Can you work these out from the model? Positions are in its coordinate system, mm. A direction names the side the tool comes from. Coordinates: 2 decimals unless noted, no trailing zeros. Order: outer loops, then holes, each group sorted by start corner. A loop starts at its lowest first (then second) coordinate and runs counter-clockwise, first axis right, second up. Notation, with made-up numbers: (85.25, 62.5) -> (122.25, 62.5) arc R30 cw to (122.25, 97.5) -> close; hole circle Ø6 at (9, 69). An arc over 180 degrees is marked (long way). Answer as a JSON object with one key per item and string values. Group by question number.
(1) I want a section at A-A, the plane x = -22. List the corners of the cut face in (y, z) for me.
(2) I need wall thicknesses on line 1 (X direction, y = 1, z = -5); line 2 (Y direction, x = -14, z = -10); line 3 (Z direction, x = 0, y = -1). Which ranges of each line are inside material? Lowest first, please.
(3) I want a section at D-D, the plane x = -47.5. List the corners of the cut face in (y, z) for me.
(4) Which directions (+Z, -Z, +X, -X, +Y, -Y) give clear straight access to the entire face, cutting with the end or side of a thin tool? Please do faces 5 (the flat face through (10.2, 1.844, 42.9)), 6 (the flat face through (7.5, 4.425, 44.7)), 7 (the flat face through (-37, -24.335, -13)), 8 (the flat face through (10.3, -4.425, 40.2)).
(5) For pin 1 (12 mm diameter, centred on x = -36, y = 27, fed in from +Z); pin 2 (3 mm diameter, centred on y = 27, z = -9, fed in from +X); pin 3 (2 mm diameter, centred on x = 11, z = 38, fed in from +Y); pin 4 (8 mm diameter, centred on y = -11, z = 5, fed in from +X), each with a flat end and sliding along its axis, tell me the tip position at first contact or that it passes through.
(6) I want a section at B-B, the plane y = -11. List the corners of the cut face in (x, z) for me.
(7) I want a section at C-C, the plane z = -18.5. List the corners of the cut face in (x, y) for me, plus the area to 3 significant figures.
(8) If we mould it in two halves opening along X, with no side actions, what happens to faces 1 (the flat face through (-29, 41.295, -13)), 2 (the cylindrical face through (11.815, -0.026, 46.62)), 3 (the flat face through (10.14, 0, -13)), 4 (the flat face through (-68.027, 0, -13))? For each: pulls with the +X half, pulls with the -X half, needs draft (parallel to the pull), parting line crosses it, or undercut.
from build123d import *

# Parameters (mm, degrees)
F0_W     = 14.748384
F0_H     = 8.849032
F0_W_2   = 7.005484
F0_H_2   = 3.687096
F3_W     = 78.166454
F3_H     = 82.406614
F3_W_2   = 44.982581
F3_H_2   = 48.669678
F4_DEPTH = 25.4
F5_DEPTH = 2.54


with BuildPart() as f2:
    # F2: sweep along a path in F1
    with BuildLine(Plane.XZ) as f2_path:
        ThreePointArc((0, 27.558451), (-16.169621, 43.728072), (-32.339242, 27.558451))
    # F0 (on Top) → F2 (sweep)
    with BuildSketch(Plane.XY):
        Rectangle(F0_W, F0_H)
        Rectangle(F0_W_2, F0_H_2, mode=Mode.SUBTRACT)
    sweep(path=f2_path.line)

    # F3 (on Top) → F4 (join)
    with BuildSketch(Plane.XY):
        with Locations((-28.943711, 0.092177)):
            Rectangle(F3_W, F3_H)
        with Locations((-36.317903, 0)):
            Rectangle(F3_W_2, F3_H_2, mode=Mode.SUBTRACT)
    extrude(amount=-F4_DEPTH)

    # F3 (on Top) → F5 (cut)
    with BuildSketch(Plane.XY):
        with Locations((-36.317903, 0)):
            Rectangle(F3_W_2, F3_H_2)
    extrude(amount=-F5_DEPTH, mode=Mode.SUBTRACT)


solid = f2.part
Computed values:
{
 "1": {"outline": "(-41.11, -25.4) -> (-24.33, -25.4) -> (-24.33, 0) -> (-41.11, 0) -> close; (-4.42, 55.89) -> (4.42, 55.89) -> (4.42, 63.33) -> (-4.42, 63.33) -> close; (24.33, -25.4) -> (41.3, -25.4) -> (41.3, 0) -> (24.33, 0) -> close; hole (-1.84, 57.32) -> (1.84, 57.32) -> (1.84, 60.91) -> (-1.84, 60.91) -> close"},
 "2": {"line 1": "x = -68.03 to -58.81, -13.83 to 10.14", "line 2": "y = -41.11 to -24.33, 24.33 to 41.3", "line 3": "z = -25.4 to 0, 1.9 to 3.57, 51.55 to 53.22, 57.31 to 60"},
 "3": {"outline": "(-41.11, -25.4) -> (-24.33, -25.4) -> (-24.33, 0) -> (-41.11, 0) -> close; (24.33, -25.4) -> (41.3, -25.4) -> (41.3, 0) -> (24.33, 0) -> close"},
 "4": {"face 5": "none", "face 6": "+Z, +X, -X, +Y", "face 7": "+Z, -Z", "face 8": "+Z, +X, -X, -Y"},
 "5": {"pin 1": "stops at z = 0", "pin 2": "stops at x = 10.14", "pin 3": "stops at y = 4.42", "pin 4": "passes through"},
 "6": {"outline": "(-68.03, -25.4) -> (-58.81, -25.4) -> (-58.81, 0) -> (-68.03, 0) -> close; (-13.83, -25.4) -> (10.14, -25.4) -> (10.14, 0) -> (-13.83, 0) -> close"},
 "7": {"outline": "(-68.03, -41.11) -> (10.14, -41.11) -> (10.14, 41.3) -> (-68.03, 41.3) -> close; hole (-58.81, -24.33) -> (-13.83, -24.33) -> (-13.83, 24.33) -> (-58.81, 24.33) -> close", "area": "4,250 mm2"},
 "8": {"face 1": "needs draft", "face 2": "undercut", "face 3": "pulls with the +X half", "face 4": "pulls with the -X half"}
}
